Input: part model. Units: mm. Frame: model coordinates. Round coordinates to 2 decimals unless told otherwise and drop trailing zeros. Order: outer loops, then holes, each group sorted by start corner. A loop starts at its lowest first (then second) coordinate and runs counter-clockwise, first axis right, second up. Notation, with made-up numbers: (0, -13) -> (54, -13) arc R7 ccw to (54, -7) -> close; hole circle Ø1 at (-10, 33). An arc over 180 degrees is marked (long way). Answer as CSV lines item,"result". Start each with the question number.
1) Section query A-A, the plane z = -20. Output: boundary loops of the cut face in (x, y).
2) Line query: L1, parallel to X at y = 2.8, z = -14.5; L2, parallel to Z at x = -20, y = 2.3; L3, parallel to Z at x = -26, y = 1.75. Output: solid intervals per line, ascending.
3) First-contact query: P1, Ø3, axis at x = -0.33, z = -9.67, coming from the +Y side; P2, Ø5.5, axis at x = -35.33, z = 20.33, coming from the -Y side; P3, Ø1.5, axis at y = 1, z = -13, coming from the -X side. Flat tips, straight axial feed; report the tip coordinate or a pass-through.
4) Section query C-C, the plane x = 30.5. Output: boundary loops of the cut face in (y, z), and give its area (3 significant figures).
5) Section query B-B, the plane y = 0.7. Output: boundary loops of the cut face in (x, z), and give its area (3 significant figures).
6) Section query D-D, the plane z = 3. Output: boundary loops of the cut face in (x, y).
```python
from build123d import *

# Parameters (mm, degrees)
SKETCH_1_R      = 1.65
EXTRUDE_1_DEPTH = 3
FILLET_1_R      = 10


with BuildPart() as part:
    # 草图1 → 凸台-拉伸1 (new body)
    with BuildSketch(Plane(origin=(0, 0, 0), x_dir=(1, 0, 0), z_dir=(0, 1, 0))):
        Polygon((-40.334108275, -30.334108275), (39.665891725, -30.334108275), (39.665891725, -10.334108275), (9.665891725, -10.334108275), (9.665891725, 29.665891725), (-10.334108275, 29.665891725), (-10.334108275, -10.334108275), (-40.334108275, -10.334108275), align=None)
        with Locations(Location((-0.334108275, -0.334108275, 0), (0, 0, 270))):
            Circle(SKETCH_1_R, mode=Mode.SUBTRACT)
        with Locations(Location((-0.334108275, 9.665891725, 0), (0, 0, 270))):
            Circle(SKETCH_1_R, mode=Mode.SUBTRACT)
        with Locations(Location((-0.334108275, 19.665891725, 0), (0, 0, 270))):
            Circle(SKETCH_1_R, mode=Mode.SUBTRACT)
        with Locations(Location((-25.334108275, -20.334108275, 0), (0, 0, 270))):
            Circle(SKETCH_1_R, mode=Mode.SUBTRACT)
        with Locations(Location((-35.334108275, -20.334108275, 0), (0, 0, 270))):
            Circle(SKETCH_1_R, mode=Mode.SUBTRACT)
        with Locations(Location((24.665891725, -20.334108275, 0), (0, 0, 270))):
            Circle(SKETCH_1_R, mode=Mode.SUBTRACT)
        with Locations(Location((34.665891725, -20.334108275, 0), (0, 0, 270))):
            Circle(SKETCH_1_R, mode=Mode.SUBTRACT)
    extrude(amount=EXTRUDE_1_DEPTH)

    # 圆角1
    fillet_1_edges = [part.edges().sort_by_distance(p)[0] for p in [
        (-10.334108275, 1.5, 10.334108275),
        (9.665891725, 1.5, 10.334108275),
    ]]
    fillet(fillet_1_edges, radius=FILLET_1_R)


solid = part.part
```
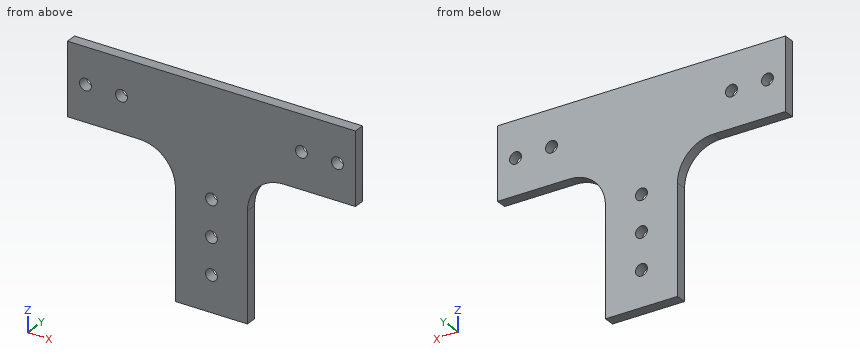
Findings:
1,outline,"(-10.33, 0) -> (-1.95, 0) -> (-1.95, 3) -> (-10.33, 3) -> close; (1.28, 0) -> (9.67, 0) -> (9.67, 3) -> (1.28, 3) -> close"
2,L1,"x = -10.33 to 9.67"
2,L2,"z = 10.33 to 30.33"
2,L3,"z = 10.33 to 18.82, 21.84 to 30.33"
3,P1,"passes through"
3,P2,"stops at y = 0"
3,P3,"stops at x = -10.33"
4,outline,"(0, 10.33) -> (3, 10.33) -> (3, 30.33) -> (0, 30.33) -> close"
4,area,"60.0 mm^2"
5,outline,"(-40.33, 10.33) -> (-20.33, 10.33) arc R10 cw to (-10.33, 0.33) -> (-10.33, -29.67) -> (9.67, -29.67) -> (9.67, 0.33) arc R10 cw to (19.67, 10.33) -> (39.67, 10.33) -> (39.67, 30.33) -> (-40.33, 30.33) -> close; hole circle Ø3.3 at (-35.33, 20.33); hole circle Ø3.3 at (-25.33, 20.33); hole circle Ø3.3 at (-0.33, -19.67); hole circle Ø3.3 at (-0.33, -9.67); hole circle Ø3.3 at (-0.33, 0.33); hole circle Ø3.3 at (24.67, 20.33); hole circle Ø3.3 at (34.67, 20.33)"
5,area,"2,380 mm^2"
6,outline,"(-10.7, 0) -> (10.03, 0) -> (10.03, 3) -> (-10.7, 3) -> close"
